The drawing under review shows one solid part. Ordinate dimensions are in mm from its lowest x, y, z. A direction names the side the tool comes from. Give positions to 0.01 mm unless a question says otherwise; leave off trailing zeros. Loops run counter-clockwise (first coordinate to the right, second up) from the corner with the lowest first, then second, coordinate; pieces in that order, holes last. Notation, with made-up numbers: (-16.75, -40) - (30.25, -40) arc R13 cw to (30.25, -26) - close; hole circle Ø3 at (-17.75, 66). An arc over 180 degrees is marked (long way). One line per item, written item: value. Start each with the question number.
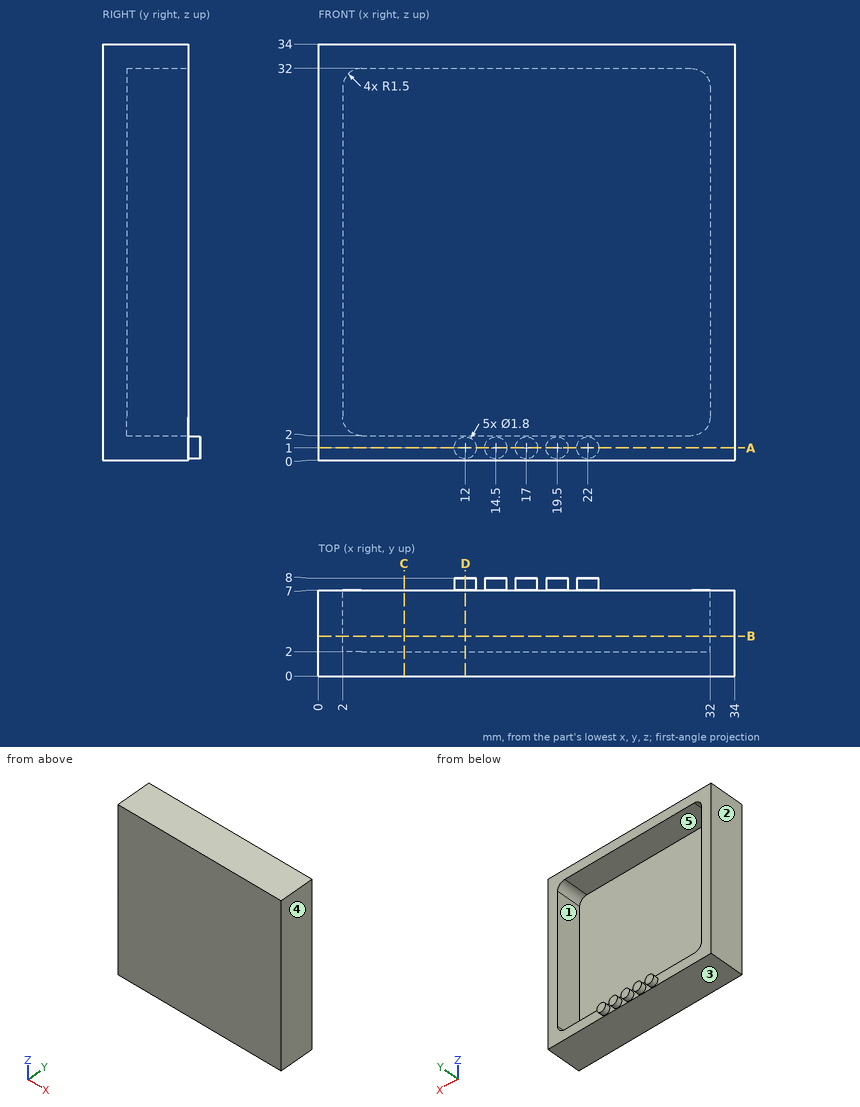
(1) Take a section at C-C on x = 7. State the section outline as (y, z) points.
(2) Take a section at D-D on x = 12. State the section outline as (y, z) points, and give its area (3 significant figures).
(3) To check wall thickness, follow L1, parallel to Z at x = 22.5, y = 2.5; L2, parallel to Y at x = 15.5, z = 29.5. State the ranges of each line that lie inside material, in increasing order. Write a range as from..to.
(4) Take a section at A-A on z = 1. State the section outline as (x, y) points, and give its area (3 significant figures).
(5) Draft analysis for pull direction X (two halves, no side actions). For the marked faces 3, 4 and 5, state which applies: pulls with the +X half, pulls with the -X half, needs draft (parallel to the pull), parting line crosses it, or undercut.
(6) For pin 1 Ø4 at (x, z) = (15.5, 15.5) entering from +Y, flat-tipped, find the tip position at first contact; note if it passes through.
(7) Machinability: for the marked faces 1 and 2, which of the approach directions +Z, -Z, +X, -X, +Y, -Y give a long, thin tool a straight path to every point of the face, cutting with its end or side? Answer none if there is none.
(8) Take a section at B-B on y = 3.25. State the section outline as (x, z) points.
Here are the results:
1. outline: (0, 0) - (7, 0) - (7, 2) - (2, 2) - (2, 32) - (7, 32) - (7, 34) - (0, 34) - close
2. outline: (0, 0) - (7, 0) - (7, 0.1) - (8, 0.1) - (8, 1.9) - (7, 1.9) - (7, 2) - (2, 2) - (2, 32) - (7, 32) - (7, 34) - (0, 34) - close
2. area: 89.8 mm²
3. L1: 0..2, 32..34
3. L2: 0..2
4. outline: (0, 0) - (34, 0) - (34, 7) - (22.9, 7) - (22.9, 8) - (21.1, 8) - (21.1, 7) - (20.4, 7) - (20.4, 8) - (18.6, 8) - (18.6, 7) - (17.9, 7) - (17.9, 8) - (16.1, 8) - (16.1, 7) - (15.4, 7) - (15.4, 8) - (13.6, 8) - (13.6, 7) - (12.9, 7) - (12.9, 8) - (11.1, 8) - (11.1, 7) - (0, 7) - close
4. area: 247 mm²
5. face 3: needs draft
5. face 4: pulls with the +X half
5. face 5: undercut
6. pin 1: y = 2
7. face 1: +Y
7. face 2: +Z, -Z, -X, +Y, -Y
8. outline: (0, 0) - (34, 0) - (34, 34) - (0, 34) - close; hole (2, 3.5) arc R1.5 ccw to (3.5, 2) - (30.5, 2) arc R1.5 ccw to (32, 3.5) - (32, 30.5) arc R1.5 ccw to (30.5, 32) - (3.5, 32) arc R1.5 ccw to (2, 30.5) - close
